```python
from build123d import *

# Parameters (mm, degrees)
SKETCH2_W           = 24
SKETCH2_H           = 8
BOSS_EXTRUDE1_DEPTH = 4
SKETCH3_R           = 1.75
CUT_EXTRUDE1_DEPTH  = 5
SKETCH4_R           = 1.45
CUT_EXTRUDE2_DEPTH  = 44
FILLET1_R           = 1


with BuildPart() as part:
    # Sketch2 → Boss-Extrude1 (new body)
    with BuildSketch(Plane.XY):
        with Locations((6.957345972, 0)):
            Rectangle(SKETCH2_W, SKETCH2_H)
    extrude(amount=BOSS_EXTRUDE1_DEPTH)

    # Sketch3 → Cut-Extrude1 (cut)
    with BuildSketch(Plane.XY.offset(4)):
        with Locations((6.957345972, 0)):
            Circle(SKETCH3_R)
    extrude(amount=-CUT_EXTRUDE1_DEPTH, mode=Mode.SUBTRACT)

    # Sketch4 → Cut-Extrude2 (cut)
    with BuildSketch(Plane.ZY.offset(5.042654028)):
        with Locations((4, 0)):
            Circle(SKETCH4_R)
    extrude(amount=-CUT_EXTRUDE2_DEPTH, mode=Mode.SUBTRACT)

    # Fillet1
    fillet1_edges = [part.edges().sort_by_distance(p)[0] for p in [
        (6.957345972, 4, 0),
        (6.957345972, -4, 0),
    ]]
    fillet(fillet1_edges, radius=FILLET1_R)


solid = part.part
```
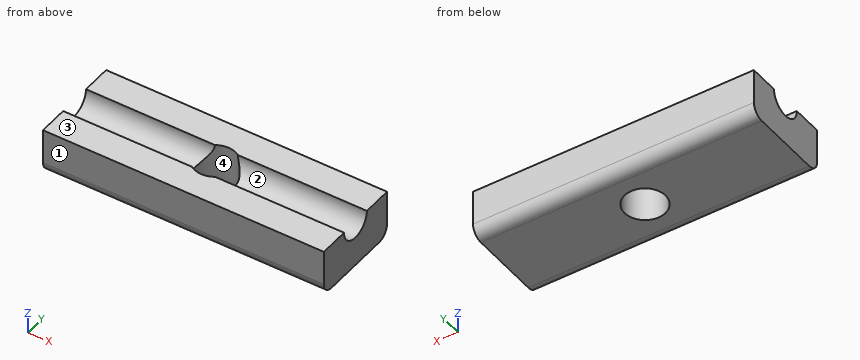
Geometry: final body of the model. Coordinates: model frame, mm. Face numbers are marked on the shaded views. Round coordinates to 2 decimals unless told otherwise and drop trailing zeros. Loops run counter-clockwise (first coordinate to the right, second up) from the corner with the lowest first, then second, coordinate; pieces in that order, holes last.
Item 1: Section B-B, the plane x = -0.75. Output: boundary loops of the cut face in (y, z).
Checked values:
outline: (-4, 1) arc R1 ccw to (-3, 0) - (3, 0) arc R1 ccw to (4, 1) - (4, 4) - (1.45, 4) arc R1.45 cw to (-1.45, 4) - (-4, 4) - close
Item 2: Line query: L1, parallel to X at y = 0, z = 2.05; L2, parallel to X at y = -0.75, z = 1.2; L3, parallel to Y at x = 9.75, z = 2.95. Output: solid intervals per line, ascending.
Checked values:
L1: x = -5.04 to 5.21, 8.71 to 18.96
L2: x = -5.04 to 5.38, 8.54 to 18.96
L3: y = -4 to -1, 1 to 4
Item 3: Mould query, pull axis Y, two halves, no side actions, for the marked faces 1, 2, 3 and 4. Classes: released by +Y, released by -Y, zero draft, split by the parting line, or undercut.
Checked values:
face 1: released by -Y
face 2: undercut
face 3: zero draft
face 4: undercut
Item 4: Section D-D, the plane z = 0.75. Output: boundary loops of the cut face in (x, y).
Checked values:
outline: (-5.04, -3.97) - (18.96, -3.97) - (18.96, 3.97) - (-5.04, 3.97) - close; hole circle Ø3.5 at (6.96, 0)
Item 5: Section A-A, the plane y = 0. Output: boundary loops of the cut face in (x, z), plus the area to 3 significant figures.
Checked values:
outline: (-5.04, 0) - (5.21, 0) - (5.21, 2.55) - (-5.04, 2.55) - close; (8.71, 0) - (18.96, 0) - (18.96, 2.55) - (8.71, 2.55) - close
area: 52.3 mm2
Item 6: Section C-C, the plane x = 6.5. Output: boundary loops of the cut face in (y, z), plus the area to 3 significant figures.
Checked values:
outline: (-4, 1) arc R1 ccw to (-3, 0) - (-1.69, 0) - (-1.69, 4) - (-4, 4) - close; (1.69, 0) - (3, 0) arc R1 ccw to (4, 1) - (4, 4) - (1.69, 4) - close
area: 18.1 mm2
